```python
from build123d import *

# Parameters (mm, degrees)
EXTRUDE_1_DEPTH     = 12
FILLET_2_R          = 2
SKETCH_2_R          = 1.55
CUT_EXTRUDE_3_DEPTH = 12
SKETCH_3_R          = 3.25
CUT_EXTRUDE_4_DEPTH = 29.62434104


with BuildPart() as part:
    # Эскиз1 → Бобышка-Вытянуть1 (new body)
    with BuildSketch(Plane.XY):
        with BuildLine():
            Line((-14, -28), (-19, -28))
            Line((-19, -28), (-19, -33))
            Line((-19, -33), (-10, -33))
            Line((-10, -33), (-10, -35.361406616))
            ThreePointArc((-10, -35.361406616), (0, -38.5), (10, -35.361406616))
            Line((10, -35.361406616), (10, -33))
            Line((10, -33), (19, -33))
            Line((19, -33), (19, -28))
            Line((19, -28), (14, -28))
            Line((14, -28), (12.5, -28))
            Line((12.5, -28), (10.356157589, -28))
            ThreePointArc((10.356157589, -28), (0, -33.5), (-10.356157589, -28))
            Line((-10.356157589, -28), (-14, -28))
        make_face()
    extrude(amount=-EXTRUDE_1_DEPTH)

    # Скругление2
    fillet_2_edges = [part.edges().sort_by_distance(p)[0] for p in [
        (-19, -30.5, 0),
        (19, -30.5, 0),
        (-10, -33, -6),
        (-10.356157589, -28, -6),
        (10.356157589, -28, -6),
        (10, -33, -6),
        (19, -30.5, -12),
        (-19, -30.5, -12),
    ]]
    fillet(fillet_2_edges, radius=FILLET_2_R)

    # Эскиз2 → Вырез-Вытянуть3 (cut)
    with BuildSketch(Plane.XZ.offset(33)):
        with Locations(Location((15.75, -6, 0), (0, 0, 270))):
            Circle(SKETCH_2_R)
        with Locations(Location((-15.75, -6, 0), (0, 0, 270))):
            Circle(SKETCH_2_R)
    extrude(amount=-CUT_EXTRUDE_3_DEPTH, mode=Mode.SUBTRACT)

    # Эскиз3 → Вырез-Вытянуть4 (cut, through all)
    with BuildSketch(Plane(origin=(0, -20.77, 0), x_dir=(1, 0, 0), z_dir=(0, 1, 0))):
        with Locations((10.5, 6)):
            Circle(SKETCH_3_R)
        with BuildLine():
            Line((0, 9.25), (0, 2.75))
            Line((0, 2.75), (10.5, 2.75))
            ThreePointArc((10.5, 2.75), (7.25, 6), (10.5, 9.25))
            Line((10.5, 9.25), (0, 9.25))
        make_face()
        with BuildLine():
            Line((-10.5, 2.75), (0, 2.75))
            Line((0, 2.75), (0, 9.25))
            Line((0, 9.25), (-10.5, 9.25))
            ThreePointArc((-10.5, 9.25), (-8.201902961, 8.298097039), (-7.25, 6))
            ThreePointArc((-7.25, 6), (-8.201902961, 3.701902961), (-10.5, 2.75))
        make_face()
        with Locations((-10.5, 6)):
            Circle(SKETCH_3_R)
    extrude(amount=-CUT_EXTRUDE_4_DEPTH, mode=Mode.SUBTRACT)


solid = part.part
```
Geometry check sheet. Reference: the model listing, model coordinates, mm. A direction names the side the tool comes from. Round coordinates to 2 decimals unless told otherwise and drop trailing zeros. Order: outer loops, then holes, each group sorted by start corner. A loop starts at its lowest first (then second) coordinate and runs counter-clockwise, first axis right, second up. Notation, with made-up numbers: (-6.5, 83.25) -> (29.5, 83.25) arc R20 cw to (29.5, 100.25) -> close; hole circle Ø7 at (-18, 8.25). An arc over 180 degrees is marked (long way). Return JSON: item names as keys, results as strings. Group by question number.
Q1. Gauge pin test, flat ends, axial feed: pin 1 (1.9 mm diameter, centred on x = 15.75, z = -6, fed in from +Y); pin 2 (6 mm diameter, centred on x = -5.5, z = -4, fed in from -Y); pin 3 (6 mm diameter, centred on x = 3.5, z = -2, fed in from -Y). Record the tip position at first contact, or that the pin passes through.
Q2. Section check D-D, the plane y = -34.5. Record the boundary of the cut face in (x, z).
Q3. Release check for a two-part mould opening along Z. For faces 1 (the flat face through (0, -34, 0)), 2 (the flat face through (0, -34, -2.75)), 3 (the cylindrical face through (-10.6, -33.57, -1.58)) record: released by +Z, released by -Z, zero draft, split by the parting line, or undercut.
Q4. Tool access check on faces 4 (the cylindrical face through (-13.75, -30.17, -6.07)), 5 (the flat face through (-14.77, -33, -4.58)), 6 (the flat face through (14, -28, -5)), 7 (the cylindrical face through (-10.5, -28.2, -1.5)), 8 (the cylindrical face through (10.57, -33.6, -1.58)). Record the directions out of +Z, -Z, +X, -X, +Y, -Y that give a thin tool (end or side, any length) a straight path to the whole face; none if there is none.
Q5. Section check A-A, the plane x = -15.75. Record the boundary of the cut face in (y, z).
Q6. Section check B-B, the plane y = -30.5. Record the boundary of the cut face in (x, z), plus the area to 3 significant figures.
Q7. Material ranges on probe 1 along X at (y, z) = (-29.75, -6); probe 2 along Z at (x, y) = (2, -35.25); probe 3 along X at (y, z) = (-32.25, -6.75), recorded low to high. Write a range as from..to.
Q8. Section check C-C, the plane z = -6. Record the boundary of the cut face in (x, y).
Numbers:
{
 "1": {"pin 1": "through", "pin 2": "y = -38.28", "pin 3": "y = -38.49"},
 "2": {"outline": "(-10.06, -12) -> (10.06, -12) -> (10.06, -9.25) -> (-10.06, -9.25) -> close; (-10.06, -2.75) -> (10.06, -2.75) -> (10.06, 0) -> (-10.06, 0) -> close"},
 "3": {"face 1": "released by +Z", "face 2": "undercut", "face 3": "zero draft"},
 "4": {"face 4": "+Y, -Y", "face 5": "+Z, -Z, -X, -Y", "face 6": "+Z, -Z, +X, -X, +Y", "face 7": "+Z, -Z, +Y", "face 8": "+Z, -Z, +X, -Y"},
 "5": {"outline": "(-33, -12) -> (-28, -12) -> (-28, -7.55) -> (-33, -7.55) -> close; (-33, -4.45) -> (-28, -4.45) -> (-28, 0) -> (-33, 0) -> close"},
 "6": {"outline": "(-19, -10) arc R2 ccw to (-17, -12) -> (-8.12, -12) -> (-8.12, -9.25) -> (-10.5, -9.25) arc R3.25 cw to (-10.5, -2.75) -> (-8.12, -2.75) -> (-8.12, 0) -> (-17, 0) arc R2 ccw to (-19, -2) -> close; (8.12, -12) -> (17, -12) arc R2 ccw to (19, -10) -> (19, -2) arc R2 ccw to (17, 0) -> (8.12, 0) -> (8.12, -2.75) -> (10.5, -2.75) arc R3.25 cw to (10.5, -9.25) -> (8.12, -9.25) -> close; hole circle Ø3.1 at (-15.75, -6); hole circle Ø3.1 at (15.75, -6)", "area": "178 mm^2"},
 "7": {"probe 1": "-19..-17.3, -14.2..-13.75, 13.75..14.2, 17.3..19", "probe 2": "-12..-9.25, -2.75..0", "probe 3": "-19..-17.11, -14.39..-13.66, 13.66..14.39, 17.11..19"},
 "8": {"outline": "(-19, -33) -> (-17.3, -33) -> (-17.3, -28) -> (-19, -28) -> close; (-14.2, -33) -> (-13.75, -33) -> (-13.75, -28) -> (-14.2, -28) -> close; (13.75, -33) -> (14.2, -33) -> (14.2, -28) -> (13.75, -28) -> close; (17.3, -33) -> (19, -33) -> (19, -28) -> (17.3, -28) -> close"}
}
